from build123d import *

# Parameters (mm, degrees)
IZIM1_R            = 15.25
IZIM1_R_2          = 12.5
TABAN_FLAN_1_DEPTH = 10


# Sheet-metal steps are written as plain solids
with BuildPart() as part:
    # Çizim1 → Taban-Flanş1 (new body)
    with BuildSketch(Plane.XY):
        with BuildLine():
            Line((29, 0), (333.542486889, 0))
            ThreePointArc((333.542486889, 0), (360, 10), (386.457513111, 0))
            Line((386.457513111, 0), (691, 0))
            ThreePointArc((691, 0), (711.506096654, -8.493903346), (720, -29))
            Line((720, -29), (720, -31))
            ThreePointArc((720, -31), (711.506096654, -51.506096654), (691, -60))
            Line((691, -60), (386.457513111, -60))
            ThreePointArc((386.457513111, -60), (360, -70), (333.542486889, -60))
            Line((333.542486889, -60), (29, -60))
            ThreePointArc((29, -60), (8.493903346, -51.506096654), (0, -31))
            Line((0, -31), (0, -29))
            ThreePointArc((0, -29), (8.493903346, -8.493903346), (29, 0))
        make_face()
        with Locations((360, -30)):
            Circle(IZIM1_R, mode=Mode.SUBTRACT)
        with Locations((695, -30)):
            Circle(IZIM1_R_2, mode=Mode.SUBTRACT)
        with Locations(Location((25, -30, 0), (0, 0, 180))):
            Circle(IZIM1_R_2, mode=Mode.SUBTRACT)
    extrude(amount=-TABAN_FLAN_1_DEPTH)


solid = part.part
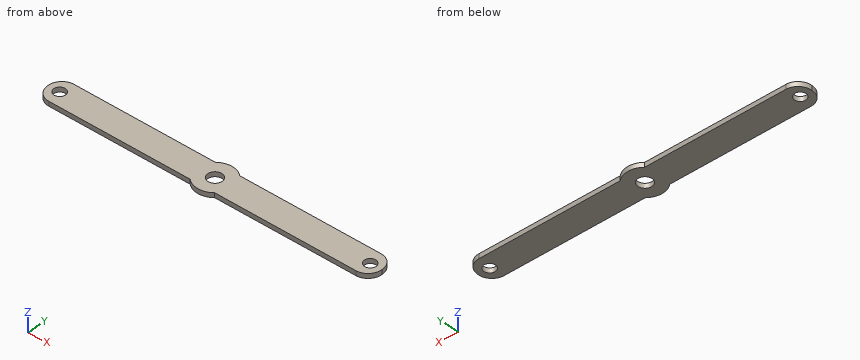
Can you work these out from the model? Positions are in its coordinate system, mm. Give positions to 0.01 mm unless a question says otherwise; leave off trailing zeros. Loops run counter-clockwise (first coordinate to the right, second up) from the corner with the lowest first, then second, coordinate; pieces in that order, holes last. Notation, with made-up numbers: (-27, 85.25) -> (0, 85.25) arc R14 cw to (0, 95.25) -> close; hole circle Ø3 at (67.5, 83). An arc over 180 degrees is marked (long way). Write item = value, one per line.
1) Suppose I cut it at A-A on x = 360. Write out the boundary of the cut face in (y, z).
Check result:
outline = (-70, -10) -> (-45.25, -10) -> (-45.25, 0) -> (-70, 0) -> close; (-14.75, -10) -> (10, -10) -> (10, 0) -> (-14.75, 0) -> close
2) Suppose I cut it at B-B on z = -7. Write out the boundary of the cut face in (x, y).
Check result:
outline = (0, -31) arc R29 ccw to (29, -60) -> (333.54, -60) arc R40 ccw to (386.46, -60) -> (691, -60) arc R29 ccw to (720, -31) -> (720, -29) arc R29 ccw to (691, 0) -> (386.46, 0) arc R40 ccw to (333.54, 0) -> (29, 0) arc R29 ccw to (0, -29) -> close; hole circle Ø25 at (25, -30); hole circle Ø30.5 at (360, -30); hole circle Ø25 at (695, -30)
3) Will these pins go through, and if not, where does the flat tip stop? pin 1 (3 mm diameter, centred on x = 496.5, z = -4, fed in from +Y); pin 2 (20 mm diameter, centred on x = 695, y = -30, fed in from +Z); pin 3 (6 mm diameter, centred on x = 309.5, z = -2, fed in from -Y).
Check result:
pin_1 = 0
pin_2 = through
pin_3 = -60
4) Suppose I cut it at C-C on x = 216. Write out the boundary of the cut face in (y, z), then the cut area to 3 significant figures.
Check result:
outline = (-60, -10) -> (0, -10) -> (0, 0) -> (-60, 0) -> close
area = 600 mm2
5) I need wall thicknesses on L1, parallel to Y at x = 288, z = -5.25; L2, parallel to Y at x = 25, z = -4.5; L3, parallel to X at y = -16.5, z = -0.5. Which ranges of each line are inside material? Lowest first, please. Write a range as from..to.
Check result:
L1 = -60..0
L2 = -59.72..-42.5, -17.5..-0.28
L3 = 2.83..352.91, 367.09..717.17
